Design review of the part built by this model. Coordinates are the model's own, in mm. A direction names the side the tool comes from. Coordinates: 2 decimals unless noted, no trailing zeros. Loops run counter-clockwise (first coordinate to the right, second up) from the corner with the lowest first, then second, coordinate; pieces in that order, holes last. Notation, with made-up numbers: (79.5, 1.5) - (92.5, 1.5) arc R25 ccw to (92.5, 19.5) - close; hole circle Ø8 at (52.5, 9). An arc over 180 degrees is marked (long way). Use one line per item in the form item = value. Start each with the question number.
(1) Add section A-A (y = 15.5). State the section outline as (x, z) points, plus the area to 3 significant figures.
(2) Tool access review of faces 1 (the face through (21, 13.95, 9)), 2 (the face through (13, -10, 4)), 3 (the face through (13, 0.1, 7)): name each direction out of +Z, -Z, +X, -X, +Y, -Y from which nothing blocks a thin tool from reaching the whole face with its end or side.
(3) Add section B-B (y = 2). State the section outline as (x, z) points, plus the area to 3 significant figures.
(4) The part is to be moulded in two halves that separate along Y. For faces 4 (the face through (13, -1.9, 4)), 5 (the face through (12.8, -4.7, -4.1)), 6 (the face through (22.6, 3.15, 0.07)), say which applies: pulls with the +Y half, pulls with the -Y half, needs draft (parallel to the pull), parting line crosses it, or undercut.
(5) Clearance check with flat-ended pins moving along their axes: pin 1 Ø0.6 at (x, y) = (4.5, 13) entering from +Z; pin 2 Ø7 at (x, z) = (21.05, 0) entering from -Y; pin 3 Ø3 at (x, z) = (21, 0.5) entering from +Y. State where each tip first meets the part, or that it passes through.
(6) For L1, parallel to Y at x = 4.75, z = 7; L2, parallel to X at y = 13, z = -7.5; L3, parallel to Z at x = 21.05, y = 14.95, list the stretches that pass through material, from the lowest coordinate up.
(7) Add section C-C (z = -1). Count the separate pieces of the cut face and the enclosed holes in it, plus the area to 3 significant figures.
Autodesk Fusion 360 part; units mm, degrees
sketch "Sketch1" plane through (0, 0, 0) normal (1, 0, 0) x (0, 1, 0)
  line L0 (-3.4393, 5.5) -> (-1.8, 5.5)
  line L1 (-12.8393, 3.9) -> (-15.5, 6.5607)
  line L2 (-7.1607, 3.9) -> (-12.8393, 3.9)
  line L3 (-4.5, 6.5607) -> (-7.1607, 3.9)
  line L4 (-4.5, -8.2) -> (-6.7372, -8.2)
  line L5 (-5.5978, 9.8222) -> (-6.8786, 8.5414)
  line L6 (-1.8, 5.5) -> (-1.8, 3.2628)
  line L7 (-19.8494, 4.4312) -> (-18.5414, 3.1214)
  line L8 (-15.5, 8.2) -> (-13.2628, 8.2)
  arc A0 (-5.1686, 10) -> (-5.5978, 9.8222) centre (-5.1686, 9.3929) ccw
  circle A1 centre (-10, 0) radius 2.1
  line L9 (-0.5, 10) -> (-5.1686, 10)
  line L10 (-6.1, 2.8393) -> (-3.4393, 5.5)
  line L11 (-14.8314, 10) -> (-19.5, 10)
  line L12 (0, -9.5) -> (0, -4.8314)
  line L13 (-15.5, -8.2) -> (-15.5, -6.5607)
  line L14 (-15.5, -6.5607) -> (-12.8393, -3.9)
  line L15 (-14.4022, -9.8222) -> (-13.1214, -8.5414)
  line L16 (-19.9987, -4.7917) -> (-20, -9.5)
  line L17 (-18.5414, -3.1214) -> (-19.8222, -4.4022)
  line L18 (-6.8786, -8.5414) -> (-5.7664, -9.6536)
  arc A2 (-19.8222, -4.4022) -> (-19.9987, -4.7917) centre (-19.3929, -4.8314) ccw
  line L19 (-13.9, -2.8393) -> (-16.5607, -5.5)
  line L20 (-16.5607, -5.5) -> (-18.2, -5.5)
  arc A3 (-0.5, -10) -> (0, -9.5) centre (-0.5, -9.5) ccw
  arc A4 (-18.2, -3.2628) -> (-18.5414, -3.1214) centre (-18.4, -3.2628) ccw
  line L21 (-13.2628, -8.2) -> (-15.5, -8.2)
  line L22 (-0.1778, -4.4022) -> (-1.4586, -3.1214)
  arc A5 (-5.7664, -9.6536) -> (-5.1686, -10) centre (-5.1163, -9.2207) ccw
  arc A6 (-20, -9.5) -> (-19.5, -10) centre (-19.5, -9.5) ccw
  line L23 (-1.8, -5.5) -> (-3.4393, -5.5)
  line L24 (-5.1686, -10) -> (-0.5, -10)
  line L25 (-3.4393, -5.5) -> (-6.1, -2.8393)
  line L26 (-12.8393, -3.9) -> (-7.1607, -3.9)
  line L27 (-4.5, -6.5607) -> (-4.5, -8.2)
  arc A7 (0, -4.8314) -> (-0.1778, -4.4022) centre (-0.6071, -4.8314) ccw
  arc A8 (-14.8314, -10) -> (-14.4022, -9.8222) centre (-14.8314, -9.3929) ccw
  line L28 (-18.2, -5.5) -> (-18.2, -3.2628)
  arc A9 (-13.1214, -8.5414) -> (-13.2628, -8.2) centre (-13.2628, -8.4) ccw
  arc A10 (-20, 4.9) -> (-19.8494, 4.4312) centre (-19.3734, 4.8428) ccw
  arc A11 (-13.2628, 8.2) -> (-13.1214, 8.5414) centre (-13.2628, 8.4) ccw
  line L29 (-13.1214, 8.5414) -> (-14.4312, 9.8494)
  arc A12 (-6.8786, 8.5414) -> (-6.7372, 8.2) centre (-6.7372, 8.4) ccw
  arc A13 (-18.5414, 3.1214) -> (-18.2, 3.2628) centre (-18.4, 3.2628) ccw
  arc A14 (-14.4312, 9.8494) -> (-14.8314, 10) centre (-14.8314, 9.3929) ccw
  line L30 (-1.4586, 3.1214) -> (-0.1778, 4.4022)
  line L31 (-15.5, 6.5607) -> (-15.5, 8.2)
  arc A15 (-19.5, 10) -> (-20, 9.5) centre (-19.5, 9.5) ccw
  arc A16 (0, 9.5) -> (-0.5, 10) centre (-0.5, 9.5) ccw
  line L32 (-20, 9.5) -> (-20, 4.9)
  line L33 (-19.5, -10) -> (-14.8314, -10)
  line L34 (-7.1607, -3.9) -> (-4.5, -6.5607)
  line L35 (-1.8, -3.2628) -> (-1.8, -5.5)
  arc A17 (-1.4586, -3.1214) -> (-1.8, -3.2628) centre (-1.6, -3.2628) ccw
  arc A18 (-6.7372, -8.2) -> (-6.8786, -8.5414) centre (-6.7372, -8.4) ccw
  arc A19 (-1.8, 3.2628) -> (-1.4586, 3.1214) centre (-1.6, 3.2628) ccw
  line L36 (0, 4.8314) -> (0, 9.5)
  line L37 (-18.2, 5.5) -> (-16.5607, 5.5)
  line L38 (-13.9, 2.8393) -> (-13.9, -2.8393)
  line L39 (-6.1, -2.8393) -> (-6.1, 2.8393)
  line L40 (-18.2, 3.2628) -> (-18.2, 5.5)
  arc A20 (-0.1778, 4.4022) -> (0, 4.8314) centre (-0.6071, 4.8314) ccw
  line L41 (-4.5, 8.2) -> (-4.5, 6.5607)
  line L42 (-6.7372, 8.2) -> (-4.5, 8.2)
  line L43 (-16.5607, 5.5) -> (-13.9, 2.8393)
  line L44 (-12.7979, 4) -> (-15.4, 6.6021)
  line L45 (-15.4, 6.6021) -> (-15.4, 8.1)
  line L46 (-15.4, 8.1) -> (-13.2628, 8.1)
  arc A21 (-13.2628, 8.1) -> (-13.0509, 8.6124) centre (-13.2628, 8.4) ccw
  line L47 (-13.0509, 8.6124) -> (-14.3627, 9.9223)
  arc A22 (-14.3627, 9.9223) -> (-14.8314, 10.1) centre (-14.8314, 9.3929) ccw
  line L48 (-14.8314, 10.1) -> (-19.5, 10.1)
  arc A23 (-19.5, 10.1) -> (-20.1, 9.5) centre (-19.5, 9.5) ccw
  line L49 (-20.1, 9.5) -> (-20.1, 4.9044)
  arc A24 (-20.1, 4.9044) -> (-19.9226, 4.363) centre (-19.3734, 4.8428) ccw
  line L50 (-19.9226, 4.363) -> (-18.6124, 3.0509)
  arc A25 (-18.6124, 3.0509) -> (-18.1, 3.2628) centre (-18.4, 3.2628) ccw
  line L51 (-18.1, 3.2628) -> (-18.1, 5.4)
  line L52 (-18.1, 5.4) -> (-16.6021, 5.4)
  line L53 (-16.6021, 5.4) -> (-14, 2.7979)
  line L54 (-14, 2.7979) -> (-14, -2.7979)
  line L55 (-14, -2.7979) -> (-16.6021, -5.4)
  line L56 (-16.6021, -5.4) -> (-18.1, -5.4)
  line L57 (-18.1, -5.4) -> (-18.1, -3.2628)
  arc A26 (-18.1, -3.2628) -> (-18.6121, -3.0507) centre (-18.4, -3.2628) ccw
  line L58 (-18.6121, -3.0507) -> (-19.8929, -4.3315)
  arc A27 (-19.8929, -4.3315) -> (-20.0987, -4.7886) centre (-19.3929, -4.8314) ccw
  line L59 (-20.0987, -4.7886) -> (-20.1, -9.4997)
  arc A28 (-20.1, -9.4997) -> (-19.5, -10.1) centre (-19.5, -9.5) ccw
  line L60 (-19.5, -10.1) -> (-14.8314, -10.1)
  arc A29 (-14.8314, -10.1) -> (-14.3315, -9.8929) centre (-14.8314, -9.3929) ccw
  line L61 (-14.3315, -9.8929) -> (-13.0507, -8.6121)
  arc A30 (-13.0507, -8.6121) -> (-13.2628, -8.1) centre (-13.2628, -8.4) ccw
  line L62 (-13.2628, -8.1) -> (-15.4, -8.1)
  line L63 (-15.4, -8.1) -> (-15.4, -6.6021)
  line L64 (-15.4, -6.6021) -> (-12.7979, -4)
  line L65 (-12.7979, -4) -> (-7.2021, -4)
  line L66 (-7.2021, -4) -> (-4.6, -6.6021)
  line L67 (-4.6, -6.6021) -> (-4.6, -8.1)
  line L68 (-4.6, -8.1) -> (-6.7372, -8.1)
  arc A31 (-6.7372, -8.1) -> (-6.9493, -8.6121) centre (-6.7372, -8.4) ccw
  line L69 (-6.9493, -8.6121) -> (-5.8439, -9.7175)
  arc A32 (-5.8439, -9.7175) -> (-5.1718, -10.1) centre (-5.1163, -9.2207) ccw
  line L70 (-5.1718, -10.1) -> (-0.5, -10.1)
  arc A33 (-0.5, -10.1) -> (0.1, -9.5) centre (-0.5, -9.5) ccw
  line L71 (0.1, -9.5) -> (0.1, -4.8314)
  arc A34 (0.1, -4.8314) -> (-0.1071, -4.3315) centre (-0.6071, -4.8314) ccw
  line L72 (-0.1071, -4.3315) -> (-1.3879, -3.0507)
  arc A35 (-1.3879, -3.0507) -> (-1.9, -3.2628) centre (-1.6, -3.2628) ccw
  line L73 (-1.9, -3.2628) -> (-1.9, -5.4)
  line L74 (-1.9, -5.4) -> (-3.3979, -5.4)
  line L75 (-3.3979, -5.4) -> (-6, -2.7979)
  line L76 (-6, -2.7979) -> (-6, 2.7979)
  line L77 (-6, 2.7979) -> (-3.3979, 5.4)
  line L78 (-3.3979, 5.4) -> (-1.9, 5.4)
  line L79 (-1.9, 5.4) -> (-1.9, 3.2628)
  arc A36 (-1.9, 3.2628) -> (-1.3879, 3.0507) centre (-1.6, 3.2628) ccw
  line L80 (-1.3879, 3.0507) -> (-0.1071, 4.3315)
  arc A37 (-0.1071, 4.3315) -> (0.1, 4.8314) centre (-0.6071, 4.8314) ccw
  line L81 (0.1, 4.8314) -> (0.1, 9.5)
  arc A38 (0.1, 9.5) -> (-0.5, 10.1) centre (-0.5, 9.5) ccw
  line L82 (-0.5, 10.1) -> (-5.1686, 10.1)
  arc A39 (-5.1686, 10.1) -> (-5.6685, 9.8929) centre (-5.1686, 9.3929) ccw
  line L83 (-5.6685, 9.8929) -> (-6.9493, 8.6121)
  arc A40 (-6.9493, 8.6121) -> (-6.7372, 8.1) centre (-6.7372, 8.4) ccw
  line L84 (-6.7372, 8.1) -> (-4.6, 8.1)
  line L85 (-4.6, 8.1) -> (-4.6, 6.6021)
  line L86 (-4.6, 6.6021) -> (-7.2021, 4)
  line L87 (-7.2021, 4) -> (-12.7979, 4)
  line L88 (0, -15) -> (0, 15) construction
  line L89 (-0.5, -10) -> (0, -10)
  line L90 (0, -10) -> (26, -10)
  line L91 (26, -10) -> (26, 20)
  line L92 (26, 20) -> (0, 20)
  line L93 (-19.5, 10) -> (0, 20)
  line L94 (13, 20) -> (13, -10) construction
  point P0 (-10, 0)
  dimension "d1" = 0.1
extrude "Extrude1" add sketch "Sketch1" along normal blind 26 contours L44 L45 L46 A21 L47 A22 L48 A33 L71 A34 L72 A35 L73 L74 L75 L76 L77 L78 L79 A36 L80 A37 L81 A38 L82 A39 L83 A40 L84 L85 L86 L87 L89 L90 L91 L92 L93
sketch "Sketch2" plane through (0, 0, 20) normal (0, 0, 1) x (-1, 0, 0)
  line L0 (0, -26) -> (0, 0)
  line L1 (0, 0) -> (-26, 0)
  line L2 (-26, 0) -> (-26, -26)
  line L3 (-26, -26) -> (0, -26)
  circle A0 centre (-13, -13) radius 8.05
  circle A1 centre (-13, -13) radius 3
  line L4 (0, -13) -> (-26, -13) construction
  line L5 (-2.15, -13.95) -> (-7.75, -13.95)
  line L6 (-7.75, -13.95) -> (-7.75, -12.05)
  line L7 (-7.75, -12.05) -> (-2.15, -12.05)
  line L8 (-2.15, -12.05) -> (-2.15, -13.95)
  line L9 (-2.15, -13.95) -> (-7.75, -12.05) construction
  line L10 (-7.75, -13.95) -> (-2.15, -12.05) construction
  line L11 (-18.25, -13.95) -> (-23.85, -13.95)
  line L12 (-23.85, -13.95) -> (-23.85, -12.05)
  line L13 (-23.85, -12.05) -> (-18.25, -12.05)
  line L14 (-18.25, -12.05) -> (-18.25, -13.95)
  line L15 (-18.25, -13.95) -> (-23.85, -12.05) construction
  line L16 (-23.85, -13.95) -> (-18.25, -12.05) construction
  point P0 (-4.95, -13)
  point P1 (-21.05, -13)
  dimension "d9" = 16.1
  dimension "d15" = 6
  dimension "d18" = 5.6
  dimension "d19" = 1.9
  dimension "d20" = 5.6
  dimension "d21" = 1.9
extrude "Extrude2" cut sketch "Sketch2" against normal blind 5.1 contours A0 L5 L6 L7 | A0 L5 L6 L7 L11 L13 L14 | A0 L11 L13 L14 | A1
extrude "Extrude3" cut sketch "Sketch2" along normal blind 5.1 from surface at -30 contours A0 L5 L6 L7 | A0 L5 L6 L7 L11 L13 L14 | A0 L11 L13 L14 | A1
extrude "Extrude4" cut sketch "Sketch2" against normal blind 30 contours A1
sketch "Sketch3" plane through (0, 26, 0) normal (0, 1, 0) x (-1, 0, 0)
  line L0 (0, -10) -> (0, 20)
  line L1 (0, 20) -> (-26, 20)
  line L2 (-26, 20) -> (-26, -10)
  line L3 (-26, -10) -> (0, -10)
  line L4 (-27, 0) -> (1, 0) construction
  circle A0 centre (-13, 0) radius 8.05 construction
  circle A1 centre (-21.05, 0) radius 3
  circle A2 centre (-21.05, 0) radius 1.55
  circle A3 centre (-4.95, 0) radius 3
  circle A4 centre (-4.95, 0) radius 1.55
  dimension "d22" = 16.1
  dimension "d23" = 6
  dimension "d24" = 3.1
  dimension "d25" = 6
  dimension "d26" = 3.1
extrude "Extrude5" cut sketch "Sketch3" against normal blind 33 contours A2 | A4
extrude "Extrude6" cut sketch "Sketch3" against normal blind 10 contours A1 | A3
extrude "Extrude7" cut sketch "Sketch2" against normal blind 23 contours A0 L5 L6 L7 | A0 L5 L7 L8 | A0 L11 L13 L14 | A0 L11 L12 L13
Computed values:
q1.outline = (0, -10) - (5.35, -10) - (5.35, -4.9) - (11.34, -4.9) - (11.34, 14.9) - (5.35, 14.9) - (5.35, 20) - (0, 20) - close; (14.66, -4.9) - (20.65, -4.9) - (20.65, -10) - (26, -10) - (26, 20) - (20.65, 20) - (20.65, 14.9) - (14.66, 14.9) - close; hole circle Ø3.1 at (4.95, 0); hole circle Ø3.1 at (21.05, 0)
q1.area = 543 mm^2
q2.face_1 = +Z
q2.face_2 = -Z, +X, -X, -Y
q2.face_3 = +X, -X
q3.outline = (0, -10) - (26, -10) - (26, 20) - (0, 20) - close; hole circle Ø3.1 at (4.95, 0); hole circle Ø3.1 at (21.05, 0)
q3.area = 765 mm^2
q4.face_4 = undercut
q4.face_5 = pulls with the -Y half
q4.face_6 = needs draft
q5.pin_1 = -3
q5.pin_2 = -6
q5.pin_3 = 16
q6.L1 = -15.4 to -4.6, 0.1 to 12.05, 13.95 to 26
q6.L2 = 0 to 4.95, 21.05 to 26
q6.L3 = -10 to -1.55, 1.55 to 20
q7.separate_pieces = 3
q7.enclosed_holes = 1
q7.area = 574 mm^2
